from build123d import *

# Parameters (mm, degrees)
BOX005_W          = 10
BOX005_H          = 10
BOX005_DEPTH      = 40
BOX004_W          = 10
BOX004_H          = 10
BOX004_DEPTH      = 40
CYLINDER011_R     = 3.7
CYLINDER011_DEPTH = 36.1


with BuildPart() as cube005:
    # Box005 → Box005 (new body)
    with BuildSketch(Plane(origin=(-1.85, -5, 5), x_dir=(1, 0, 0), z_dir=(0, 0, 1))):
        with Locations((5, 5)):
            Rectangle(BOX005_W, BOX005_H)
    extrude(amount=BOX005_DEPTH)


with BuildPart() as cube004:
    # Box004 → Box004 (new body)
    with BuildSketch(Plane(origin=(13.05, -5, -11), x_dir=(1, 0, 0), z_dir=(0, 0, 1))):
        with Locations((5, 5)):
            Rectangle(BOX004_W, BOX004_H)
    extrude(amount=BOX004_DEPTH)


with BuildPart() as drive:
    # Cylinder011 → Cylinder011 (new body)
    with BuildSketch(Plane(origin=(10.6, 0, -9.2), x_dir=(1, 0, 0), z_dir=(0, 0, 1))):
        Circle(CYLINDER011_R)
    extrude(amount=CYLINDER011_DEPTH)

    # Cut005: cut Cube004
    add(cube004.part, mode=Mode.SUBTRACT)

    # Cut006: cut Cube005
    add(cube005.part, mode=Mode.SUBTRACT)


with BuildPart() as drive_1:
    # Cut006 placement: moved
    add(drive.part.moved(Location((-10.6, 0, 3))))


solid = drive_1.part
For this review, take the finished solid that the model builds, in its own axes (mm). A direction names the side the tool comes from. Coordinates: 2 decimals unless noted, no trailing zeros. Order: outer loops, then holes, each group sorted by start corner. A loop starts at its lowest first (then second) coordinate and runs counter-clockwise, first axis right, second up. Notation, with made-up numbers: (63.25, 34.25) -> (78.25, 34.25) arc R25 cw to (78.25, 49.25) -> close; hole circle Ø9 at (-2.75, 41). An arc over 180 degrees is marked (long way). Return JSON: item names as keys, results as strings.
1. We need section B-B on z = 0. Write out the cut boundary in (x, y).
Answer block:
{"outline": "(2.45, -2.77) -> (2.45, 2.77) arc R3.7 ccw (long way) to start"}
2. We need section C-C on x = -1. Write out the cut boundary in (y, z), and give its area (3 significant figures).
Answer block:
{"outline": "(-3.56, -6.2) -> (3.56, -6.2) -> (3.56, 29.9) -> (-3.56, 29.9) -> close", "area": "257 mm²"}
3. For pin 1 Ø2 at (y, z) = (-1, 15) entering from -X; pin 2 Ø1.7 at (y, z) = (-1.5, 22) entering from -X; pin 3 Ø1 at (x, y) = (-3, -0.5) entering from +Z, all flat-tipped, find the tip position at first contact; note any pin that passes through.
Answer block:
{"pin 1": "x = -2.45", "pin 2": "x = -2.45", "pin 3": "z = 8"}
4. We need section A-A on y = 0. Write out the cut boundary in (x, z), and give its area (3 significant figures).
Answer block:
{"outline": "(-3.7, -6.2) -> (2.45, -6.2) -> (2.45, 29.9) -> (-2.45, 29.9) -> (-2.45, 8) -> (-3.7, 8) -> close", "area": "195 mm²"}
5. We need section D-D on z = 25. Write out the cut boundary in (x, y), and give its area (3 significant figures).
Answer block:
{"outline": "(-2.45, -2.77) arc R3.7 ccw to (2.45, -2.77) -> (2.45, 2.77) arc R3.7 ccw to (-2.45, 2.77) -> close", "area": "33.4 mm²"}
6. Machinability: for faces 1 (the flat face through (2.45, 0, 12)), 2 (the flat face through (-2.45, 0, 19)), which of the approach directions +Z, -Z, +X, -X, +Y, -Y give a long, thin tool a straight path to every point of the face, cutting with its end or side? Answer none if there is none.
Answer block:
{"face 1": "+Z, -Z, +X, +Y, -Y", "face 2": "+Z, -X, +Y, -Y"}
7. For line 1 (X direction, y = 1.75, z = 15.5); line 2 (Z direction, x = -2.5, y = -1.5); line 3 (Y direction, x = -0.25, z = 12), list the stretches that pass through material, from the lowest coordinate up. Write a range as from..to.
Answer block:
{"line 1": "-2.45..2.45", "line 2": "-6.2..8", "line 3": "-3.69..3.69"}
